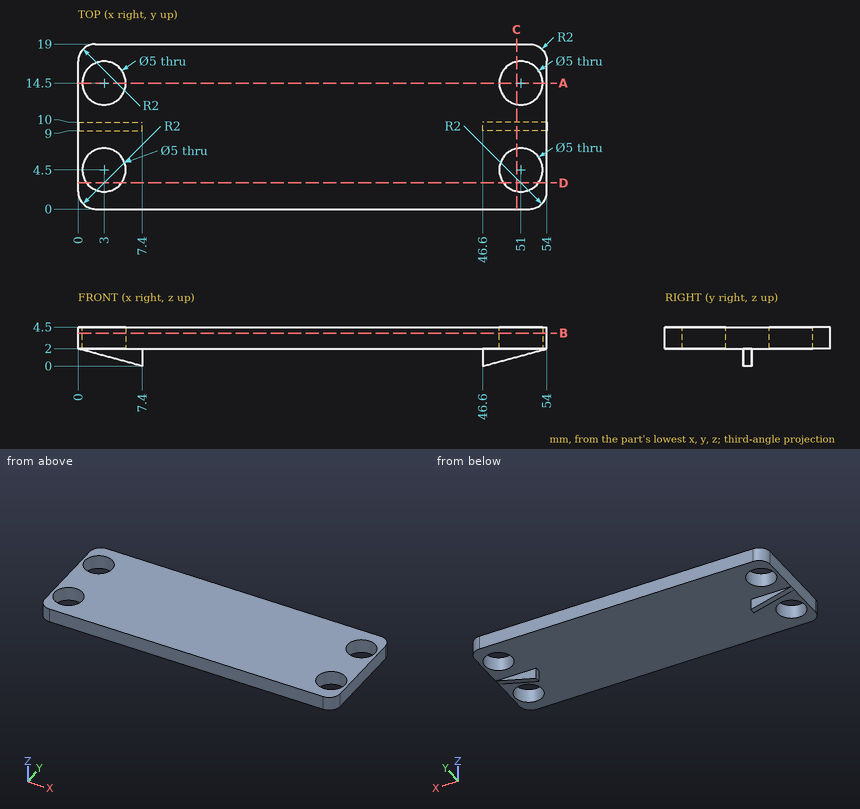
Here's the drawing with two shaded views (mm, measured from the low corner). I have some questions. Round coordinates to 2 decimals unless told otherwise and drop trailing zeros. Write each loop counter-clockwise with the first axis right and the second up, starting at its lowest first coordinate (ties: lowest second). Pieces come first, ordered by that corner, then holes. Notation, with made-up numbers: M -7.75,-6.75 L 19.25,-6.75 A11 ccw 19.25,5.25 Z; hole C 86,8 d6. An arc over 180 degrees is marked long. Write each question's results on one line, items separated by ' | '. Start each with the question number.
1. Imagine slicing it at C-C on x = 50.5. List the corners of the cut face in (y, z) for me.
2. Imagine slicing it at D-D on y = 3. List the corners of the cut face in (x, z) for me.
3. Imagine slicing it at A-A on y = 14.5. List the corners of the cut face in (x, z) for me, and give its area (3 significant figures).
4. I'm going to push flat-ended pins straight in: pin 1 Ø0.6 at (x, z) = (4, 1.5) entering from +Y; pin 2 Ø1 at (x, y) = (6.5, 15.5) entering from -Z. Where does each tip first touch, or does it pass through?
5. Imagine slicing it at B-B on z = 3.8. List the corners of the cut face in (x, y) for me.
6. I need wall thicknesses on L1, parallel to Y at x = 51, z = 2.7; L2, parallel to Y at x = 50.5, z = 2.6; L3, parallel to X at y = 13, z = 3.15. Which ranges of each line are inside material? Lowest first, please. Write a range as from..to.
Result sheet:
1) outline: M 0,2 L 2.05,2 L 2.05,4.5 L 0,4.5 Z; M 6.95,2 L 9,2 L 9,1.05 L 10,1.05 L 10,2 L 12.05,2 L 12.05,4.5 L 6.95,4.5 Z; M 16.95,2 L 19,2 L 19,4.5 L 16.95,4.5 Z
2) outline: M 0,2 L 1,2 L 1,4.5 L 0,4.5 Z; M 5,2 L 49,2 L 49,4.5 L 5,4.5 Z; M 53,2 L 54,2 L 54,4.5 L 53,4.5 Z
3) outline: M 0,2 L 0.5,2 L 0.5,4.5 L 0,4.5 Z; M 5.5,2 L 48.5,2 L 48.5,4.5 L 5.5,4.5 Z; M 53.5,2 L 54,2 L 54,4.5 L 53.5,4.5 Z | area: 110 mm^2
4) pin 1: stops at y = 10 | pin 2: stops at z = 2
5) outline: M 0,2 A2 ccw 2,0 L 52,0 A2 ccw 54,2 L 54,17 A2 ccw 52,19 L 2,19 A2 ccw 0,17 Z; hole C 3,4.5 d5; hole C 3,14.5 d5; hole C 51,4.5 d5; hole C 51,14.5 d5
6) L1: y = 0..2, 7..12, 17..19 | L2: y = 0..2.05, 6.95..12.05, 16.95..19 | L3: x = 0..1, 5..49, 53..54
